from build123d import *

# Parameters (mm, degrees)
F0_R     = 2.5
F0_R_2   = 1.5
F1_DEPTH = 1
F2_DEPTH = 64
F3_DEPTH = 1


with BuildPart() as f1:
    # F0 (on Front) → F1 (new body)
    with BuildSketch(Plane.XZ):
        Circle(F0_R)
        Circle(F0_R_2, mode=Mode.SUBTRACT)
        Circle(F0_R_2)
    extrude(amount=F1_DEPTH)

    # F0 (on Front) → F2 (join)
    with BuildSketch(Plane.XZ):
        Circle(F0_R_2)
    extrude(amount=F2_DEPTH)

    # F3 (add): a face of the model
    f3_faces = [f1.faces().sort_by_distance(p)[0] for p in [
        (0, -64, 0),
    ]]
    extrude(f3_faces, amount=F3_DEPTH)


solid = f1.part
Could you check a few things on this model? Use its own coordinates, in mm. A direction names the side the tool comes from. Give positions to 0.01 mm unless a question says otherwise; leave off trailing zeros. Order: outer loops, then holes, each group sorted by start corner. A loop starts at its lowest first (then second) coordinate and runs counter-clockwise, first axis right, second up. Notation, with made-up numbers: (-18.5, 53.5) -> (8.5, 53.5) arc R22 cw to (8.5, 85.5) -> close; hole circle Ø8 at (15.25, 32.25). An arc over 180 degrees is marked (long way). Answer in a Markdown table with one row per item. Add a question column.
Item 1: Imagine slicing it at C-C (y = -28). List the corners of the cut face in (x, z) for me.
Item 2: Please list where these lines run through material, in increasing order: probe 1 along X at (y, z) = (-18, -0.15); probe 2 along Y at (x, z) = (1.5, -0.9); probe 3 along Z at (x, y) = (0.6, -24.5).
Item 3: I'm going to push flat-ended pins straight in: P1, Ø2, axis at y = -53, z = -1, coming from the +X side; P2, Ø3, axis at x = 0.5, y = -49.5, coming from the +Z side; P3, Ø2, axis at x = -0.5, y = -55, coming from the -Z side. Where does each tip first touch, or does it pass through?
Item 4: Imagine slicing it at B-B (x = 0). List the corners of the cut face in (y, z) for me, and give its area (3 significant figures).
Item 5: Imagine slicing it at A-A (z = 0). List the corners of the cut face in (x, y) for me, and give its area (3 significant figures).
Item 6: For faces 1 (the flat face through (0, -65, 0)), 2 (the cylindrical face through (-1.5, -32.55, 0.07)), which set-ups out of +Z, -Z, +X, -X, +Y, -Y let a thin tool reach every point of the face, with its end or its side?
Result:
| question | item | result |
|---|---|---|
| 1 | outline | circle Ø3 at (0, 0) |
| 2 | probe 1 | -1.49 to 1.49 |
| 2 | probe 2 | -1 to 0 |
| 2 | probe 3 | -1.37 to 1.37 |
| 3 | P1 | x = 1.5 |
| 3 | P2 | z = 1.5 |
| 3 | P3 | z = -1.5 |
| 4 | outline | (-65, -1.5) -> (-1, -1.5) -> (-1, -2.5) -> (0, -2.5) -> (0, 2.5) -> (-1, 2.5) -> (-1, 1.5) -> (-65, 1.5) -> close |
| 4 | area | 197 mm2 |
| 5 | outline | (-2.5, -1) -> (-1.5, -1) -> (-1.5, -65) -> (1.5, -65) -> (1.5, -1) -> (2.5, -1) -> (2.5, 0) -> (-2.5, 0) -> close |
| 5 | area | 197 mm2 |
| 6 | face 1 | +Z, -Z, +X, -X, -Y |
| 6 | face 2 | -Y |
